Geometry: see drawing. Coordinates: mm, zero at the bounding-box minimum. A direction names the side the tool comes from. Give positions to 0.01 mm unless a question says otherwise; leave off trailing zeros. Loops run counter-clockwise (first coordinate to the right, second up) from the corner with the lowest first, then second, coordinate; pieces in that order, holes last. Notation, with made-up numbers: M -1,20 L 26,20 A23 ccw 26,41 Z; hole C 29.5,3 d7. An arc over 180 degrees is marked long. Answer in a Markdown table with one row per item.
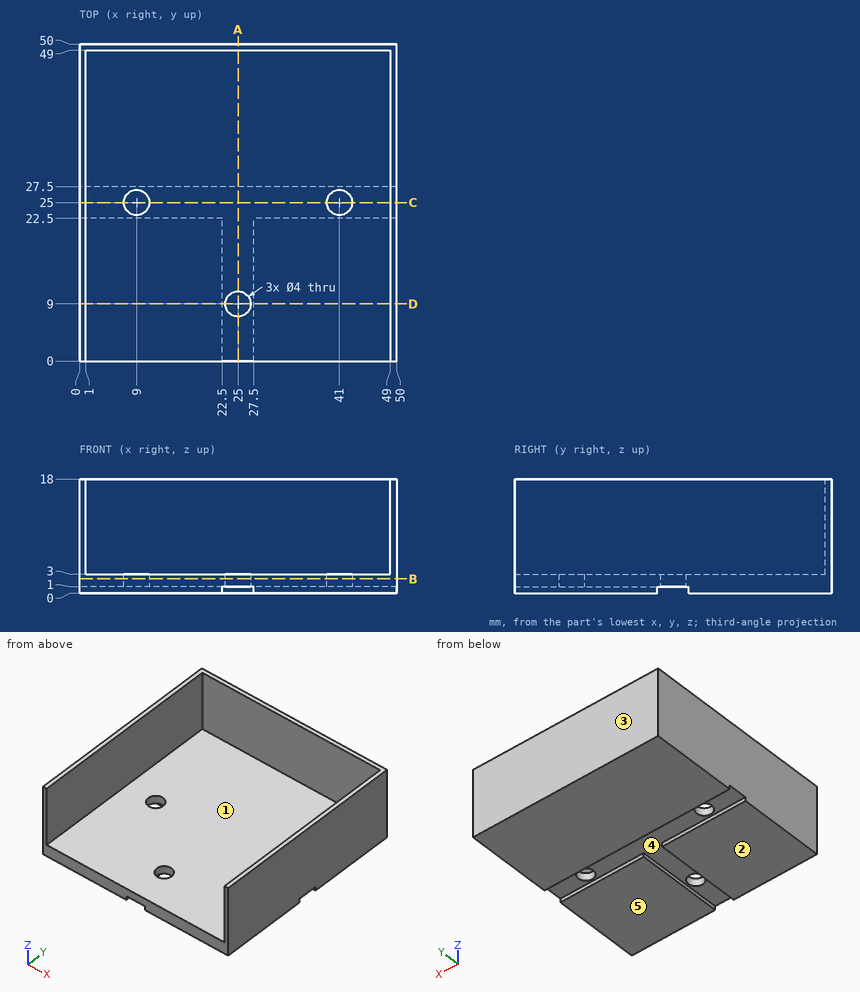
1) Material intervals for L1, parallel to X at y = 3, z = 4.25; L2, parallel to Y at x = 9, z = 2.15; L3, parallel to Y at x = 25, z = 2.3, sorted ascending.
Reply:
| item | result |
|---|---|
| L1 | x = 0 to 1, 49 to 50 |
| L2 | y = 0 to 23, 27 to 50 |
| L3 | y = 0 to 7, 11 to 50 |
2) Pin query (flat end, axial travel): pin 1 Ø5 at (x, z) = (34.5, 15) entering from -Y; pin 2 Ø2.5 at (x, y) = (41, 25) entering from -Z. Return the tip coordinate at first contact, or that it passes through.
Reply:
| item | result |
|---|---|
| pin 1 | stops at y = 49 |
| pin 2 | passes through |
3) Set-up query: the marked faces 1 and 2. Return all of +Z, -Z, +X, -X, +Y, -Y with unobstructed straight access to the full face (end or side cutting, diameter ignored); none if empty.
Reply:
| item | result |
|---|---|
| face 1 | +Z, -Y |
| face 2 | -Z, +X, -X, +Y, -Y |
4) Section B-B, the plane z = 2.25. Return loops of the section in (x, y), then the cut area to 3 significant figures.
Reply:
| item | result |
|---|---|
| outline | M 0,0 L 50,0 L 50,50 L 0,50 Z; hole C 9,25 d4; hole C 25,9 d4; hole C 41,25 d4 |
| area | 2,460 mm² |
5) Section C-C, the plane y = 25. Return loops of the section in (x, z).
Reply:
| item | result |
|---|---|
| outline | M 0,1 L 7,1 L 7,3 L 1,3 L 1,18 L 0,18 Z; M 11,1 L 39,1 L 39,3 L 11,3 Z; M 43,1 L 50,1 L 50,18 L 49,18 L 49,3 L 43,3 Z |
6) Pull-direction query (Y, two-part tool) for the marked faces 3, 4 and 5; classes: released by +Y, released by -Y, zero draft, split by the parting line, or undercut.
Reply:
| item | result |
|---|---|
| face 3 | released by +Y |
| face 4 | undercut |
| face 5 | zero draft |
7) Section A-A, the plane x = 25. Return loops of the section in (y, z), then the cut area to 4 significant figures.
Reply:
| item | result |
|---|---|
| outline | M 0,1 L 7,1 L 7,3 L 0,3 Z; M 11,1 L 27.5,1 L 27.5,0 L 50,0 L 50,18 L 49,18 L 49,3 L 11,3 Z |
| area | 129.5 mm² |
8) Section D-D, the plane y = 9. Return loops of the section in (x, z).
Reply:
| item | result |
|---|---|
| outline | M 0,0 L 22.5,0 L 22.5,1 L 23,1 L 23,3 L 1,3 L 1,18 L 0,18 Z; M 27,1 L 27.5,1 L 27.5,0 L 50,0 L 50,18 L 49,18 L 49,3 L 27,3 Z |
